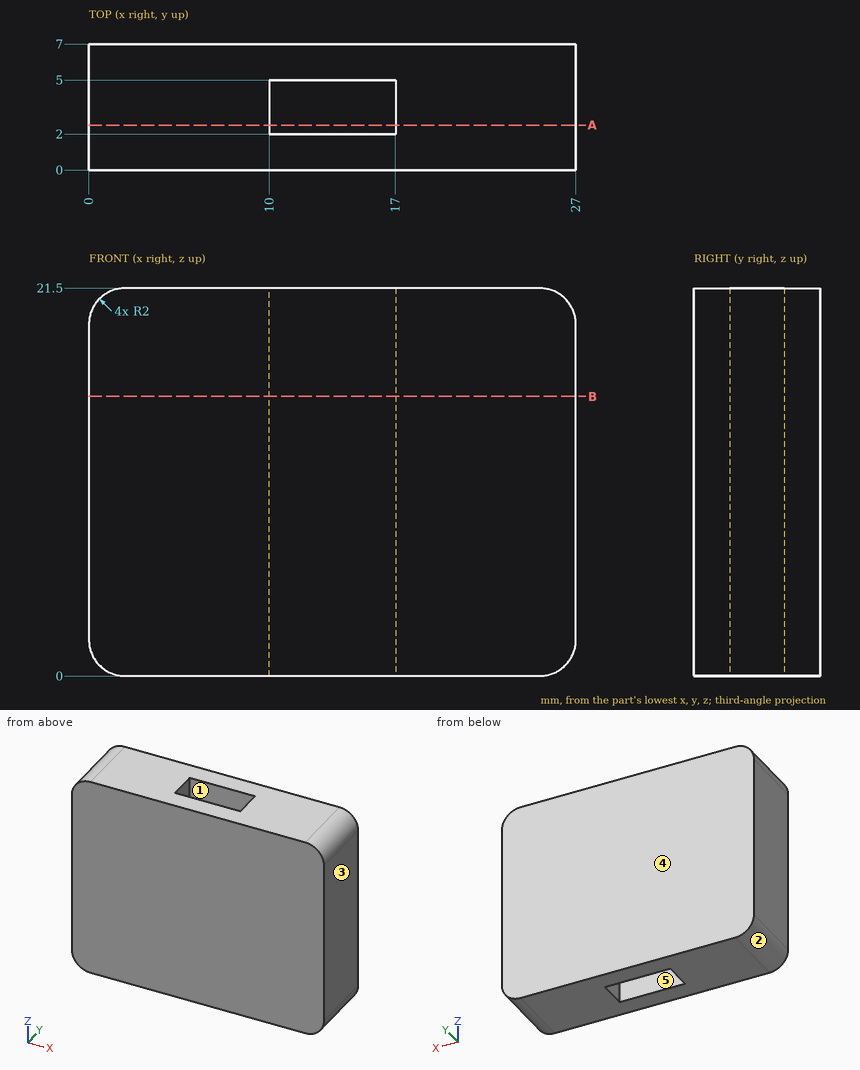
Here's the drawing with two shaded views (mm, measured from the low corner). I have some questions. A direction names the side the tool comes from. Round coordinates to 2 decimals unless told otherwise and drop trailing zeros. Loops run counter-clockwise (first coordinate to the right, second up) from the corner with the lowest first, then second, coordinate; pieces in that order, holes last. Notation, with made-up numbers: M 15,31 L 65,31 A27 cw 65,68 Z; hole C 69.25,45 d10. An arc over 180 degrees is marked long. Answer as CSV lines item,"result".
1) Imagine slicing it at A-A on y = 2.5. List the corners of the cut face in (x, z) for me.
From the geometry:
outline,"M 0,2 A2 ccw 2,0 L 10,0 L 10,21.5 L 2,21.5 A2 ccw 0,19.5 Z; M 17,0 L 25,0 A2 ccw 27,2 L 27,19.5 A2 ccw 25,21.5 L 17,21.5 Z"
2) If I drill on probe 1 along X at (y, z) = (4.5, 17); probe 2 along Y at (x, z) = (16.25, 12), over which ranges is the centre line in solid material (lowest first)?
From the geometry:
probe 1,"0 to 10, 17 to 27"
probe 2,"0 to 2, 5 to 7"
3) We'd pull the mould along X, two halves only. Please class the marked faces 3, 4 and 5: released by +X, released by -X, zero draft, split by the parting line, or undercut.
From the geometry:
face 3,"released by +X"
face 4,"zero draft"
face 5,"undercut"
4) Which directions (+Z, -Z, +X, -X, +Y, -Y) give clear straight access to the entire face, cutting with the end or side of a thin tool? Please do the marked faces 1 and 2.
From the geometry:
face 1,"+Z, -Z"
face 2,"-Z, -X, +Y, -Y"
5) Imagine slicing it at B-B on z = 15.5. List the corners of the cut face in (x, y) for me, and give its area (3 significant figures).
From the geometry:
outline,"M 0,0 L 27,0 L 27,7 L 0,7 Z; hole M 10,2 L 17,2 L 17,5 L 10,5 Z"
area,"168 mm^2"
